```python
from build123d import *

# Parameters (mm, degrees)
SKETCH1_R                = 3
BOSS_EXTRUDE1_DEPTH      = 8
CUT_EXTRUDE1_DEPTH       = 35
SKETCH4_R                = 4
BOSS_EXTRUDE2_DEPTH      = 6
CHAMFER1_SIZE            = 0.8
CHAMFER1_OF_MIRROR1_SIZE = 0.8


with BuildPart() as part:
    # Sketch1 → Boss-Extrude1 (new body)
    with BuildSketch(Plane(origin=(0, 0, 0), x_dir=(1, 0, 0), z_dir=(0, 1, 0))):
        with BuildLine():
            Line((39.626089151, 56.371006445), (-40.373910849, 56.371006445))
            ThreePointArc((-40.373910849, 56.371006445), (-50.980512566, 51.977608163), (-55.373910849, 41.371006445))
            Line((-55.373910849, 41.371006445), (-55.373910849, -38.628993555))
            ThreePointArc((-55.373910849, -38.628993555), (-50.980512566, -49.235595273), (-40.373910849, -53.628993555))
            Line((-40.373910849, -53.628993555), (39.626089151, -53.628993555))
            ThreePointArc((39.626089151, -53.628993555), (50.232690869, -49.235595273), (54.626089151, -38.628993555))
            Line((54.626089151, -38.628993555), (54.626089151, 41.371006445))
            ThreePointArc((54.626089151, 41.371006445), (50.232690869, 51.977608163), (39.626089151, 56.371006445))
        make_face()
        with Locations(Location((-48.373910849, 34.371006445, 0), (0, 0, 270))):
            Circle(SKETCH1_R, mode=Mode.SUBTRACT)
        with Locations(Location((-33.373910849, 49.371006445, 0), (0, 0, 270))):
            Circle(SKETCH1_R, mode=Mode.SUBTRACT)
        with Locations(Location((32.626089151, 49.371006445, 0), (0, 0, 270))):
            Circle(SKETCH1_R, mode=Mode.SUBTRACT)
        with Locations(Location((-48.373910849, -31.628993555, 0), (0, 0, 270))):
            Circle(SKETCH1_R, mode=Mode.SUBTRACT)
        with Locations(Location((-33.373910849, -46.628993555, 0), (0, 0, 270))):
            Circle(SKETCH1_R, mode=Mode.SUBTRACT)
        with Locations(Location((32.626089151, -46.628993555, 0), (0, 0, 270))):
            Circle(SKETCH1_R, mode=Mode.SUBTRACT)
    extrude(amount=BOSS_EXTRUDE1_DEPTH)

    # Sketch3 → Cut-Extrude1 (cut)
    with BuildSketch(Plane(origin=(54.626089151, 0, 0), x_dir=(0, 0, -1), z_dir=(1, 0, 0))):
        Polygon((-30, 8), (-30, 5.5), (-36, 5.5), (-36, 2.5), (-30, 2.5), (-30, 1.25), (30, 1.25), (30, 2.5), (36, 2.5), (36, 5.5), (30, 5.5), (30, 8), align=None)
    extrude(amount=-CUT_EXTRUDE1_DEPTH, mode=Mode.SUBTRACT)

    # Sketch4 → Boss-Extrude2 (add)
    with BuildSketch(Plane(origin=(0, 8, 0), x_dir=(1, 0, 0), z_dir=(0, 1, 0))):
        with Locations(Location((4.626089151, -38.628993555, 0), (0, 0, 270))):
            Circle(SKETCH4_R)
        with Locations(Location((-40.373910849, -38.628993555, 0), (0, 0, 270))):
            Circle(SKETCH4_R)
    boss_extrude2 = extrude(amount=BOSS_EXTRUDE2_DEPTH)

    # Chamfer1
    chamfer1_edges = [part.edges().sort_by_distance(p)[0] for p in [
        (4.626089151, 14, 34.628993555),
        (-40.373910849, 14, 34.628993555),
    ]]
    chamfer(chamfer1_edges, length=CHAMFER1_SIZE)

    # Mirror1: Boss-Extrude2 across plane
    add(boss_extrude2.mirror(Plane.XY))

    # Chamfer1 of Mirror1
    chamfer1_of_mirror1_edges = [part.edges().sort_by_distance(p)[0] for p in [
        (4.626089151, 14, -34.628993555),
        (-40.373910849, 14, -34.628993555),
    ]]
    chamfer(chamfer1_of_mirror1_edges, length=CHAMFER1_OF_MIRROR1_SIZE)


solid = part.part
```
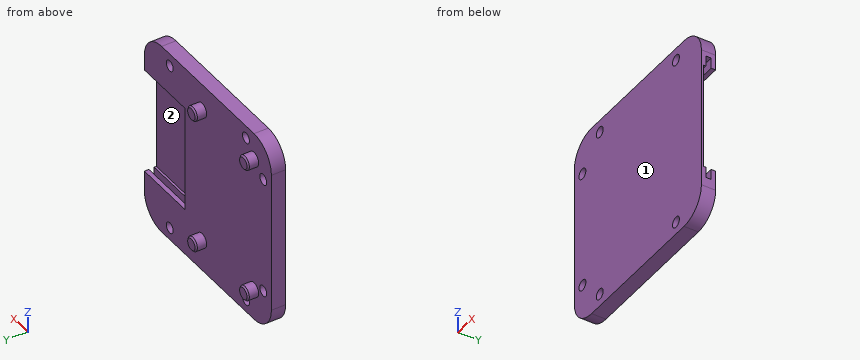
Work out the finished part from the listing and answer in its coordinate system (mm). Face numbers are marked on the shaded views. A direction names the side the tool comes from. Give positions to 0.01 mm unless a question says otherwise; leave off trailing zeros. Write each loop counter-clockwise with the first axis right and the second up, starting at its lowest first coordinate (ties: lowest second). Pieces come first, ordered by that corner, then holes. Notation, with made-up numbers: (-24, 66.5) - (8, 66.5) arc R18 cw to (8, 84.5) - close; hole circle Ø4 at (31.5, 3.25). An arc over 180 degrees is marked (long way). Use one line per item in the form item = value.
1. A cutting plane is placed at A-A (z = 5). Write down the section's boundary in (x, y), and give its area (3 significant figures).
Filled in:
outline = (-55.37, 0) - (54.63, 0) - (54.63, 1.25) - (19.63, 1.25) - (19.63, 8) - (-55.37, 8) - close
area = 644 mm^2
2. A cutting plane is placed at B-B (y = 9.75). Write down the section's boundary in (x, z).
Filled in:
outline = circle Ø8 at (-40.37, -38.63); circle Ø8 at (-40.37, 38.63); circle Ø8 at (4.63, -38.63); circle Ø8 at (4.63, 38.63)
3. Each of these flat-tipped pins is pushed along its axis until it touches: pin 1 Ø9.5 at (x, z) = (-48.37, 31.63) entering from +Y; pin 2 Ø1.5 at (y, z) = (7.5, -2.5) entering from +X; pin 3 Ø1 at (x, y) = (42, 1.5) entering from +Z; pin 4 Ø5.5 at (x, z) = (-48.37, -34.37) entering from -Y. Where does it stop, or does it pass through?
Filled in:
pin_1 = 8
pin_2 = 19.63
pin_3 = 53.51
pin_4 = through
4. Consider L1, parallel to Z at x = 38.5, y = 3.75; L2, parallel to Y at x = 36.5, z = -31.5; L3, parallel to X at y = 1.75, z = -50.5. Determine where each line is inside the solid, lowest interval first.
Filled in:
L1 = -56.37 to -36, 36 to 53.63
L2 = 0 to 2.5, 5.5 to 8
L3 = -52.28 to -36.15, -30.59 to 29.85, 35.41 to 51.53
5. For the marked faces 1 and 2, determine the directions among +Z, -Z, +X, -X, +Y, -Y from which every point of the face is accessible in a straight line to the end or side of a thin tool.
Filled in:
face_1 = +Z, -Z, +X, -X, -Y
face_2 = +X, +Y
6. A cutting plane is placed at C-C (x = 16). Write down the section's boundary in (y, z).
Filled in:
outline = (0, -56.37) - (8, -56.37) - (8, 53.63) - (0, 53.63) - close
